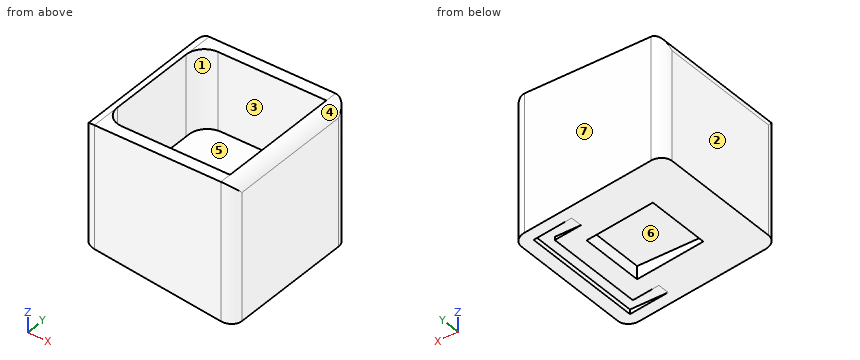
from build123d import *

# Parameters (mm, degrees)
F0_W     = 25
F0_H     = 25
F0_W_2   = 21
F0_H_2   = 21
F1_DEPTH = 23
F0_W_3   = 17
F0_H_3   = 17
F2_DEPTH = 5
F0_W_4   = 11
F0_H_4   = 11
F3_DEPTH = 12
F4_DEPTH = 3
F5_DEPTH = 1
F7_DEPTH = 25
F8_R     = 1.99999
F9_R     = 3


# Not quite as in the source:
# - a fillet or chamfer is up to 0.001 mm smaller than in the source, because OpenCascade refuses the exact size


with BuildPart() as f1:
    # F0 (on Top) → F1 (new body)
    with BuildSketch(Plane.XY):
        with Locations((12.5, -12.5)):
            Rectangle(F0_W, F0_H)
        with Locations((12.5, -12.5)):
            Rectangle(F0_W_2, F0_H_2, mode=Mode.SUBTRACT)
    extrude(amount=F1_DEPTH)

    # F0 (on Top) → F2 (join)
    with BuildSketch(Plane.XY):
        with Locations((12.5, -12.5)):
            Rectangle(F0_W_2, F0_H_2)
        with Locations((12.5, -12.5)):
            Rectangle(F0_W_3, F0_H_3, mode=Mode.SUBTRACT)
    extrude(amount=F2_DEPTH)

    # F0 (on Top) → F3 (join)
    with BuildSketch(Plane.XY):
        with Locations((12.5, -12.5)):
            Rectangle(F0_W_3, F0_H_3)
        with Locations((12.5, -12.5)):
            Rectangle(F0_W_4, F0_H_4, mode=Mode.SUBTRACT)
        with Locations((12.5, -12.5)):
            Rectangle(F0_W_4, F0_H_4)
    extrude(amount=F3_DEPTH)

    # F0 (on Top) → F4 (cut)
    with BuildSketch(Plane.XY):
        with Locations((12.5, -12.5)):
            Rectangle(F0_W_4, F0_H_4)
    extrude(amount=F4_DEPTH, mode=Mode.SUBTRACT)

    # F0 (on Top) → F5 (cut)
    with BuildSketch(Plane.XY):
        with Locations((12.5, -12.5)):
            Rectangle(F0_W_2, F0_H_2)
        with Locations((12.5, -12.5)):
            Rectangle(F0_W_3, F0_H_3, mode=Mode.SUBTRACT)
    extrude(amount=F5_DEPTH, mode=Mode.SUBTRACT)

    # F6 (on face) → F7 (cut, through all)
    with BuildSketch(Plane.XZ.offset(25)):
        Polygon((25, 0), (0, 3), (0, 0), align=None)
    extrude(amount=-F7_DEPTH, mode=Mode.SUBTRACT)

    # F8 (radius 2 in the source; OpenCascade refuses exactly that, so slightly less here)
    f8_edges = [f1.edges().sort_by_distance(p)[0] for p in [
        (25, -25, 11.5),
        (0, -25, 13),
        (0, 0, 13),
        (25, 0, 11.5),
        (0, -12.5, 23),
        (25, -12.5, 23),
    ]]
    fillet(f8_edges, radius=F8_R)

    # F9
    f9_edges = [f1.edges().sort_by_distance(p)[0] for p in [
        (2, -2, 14),
        (4, -4, 8.5),
        (21, -4, 8.5),
        (21, -21, 8.5),
        (4, -21, 8.5),
        (2, -23, 14),
    ]]
    fillet(f9_edges, radius=F9_R)


solid = f1.part
Geometry check sheet. Reference: the model listing, model coordinates, mm. Face numbers are marked on the shaded views. A direction names the side the tool comes from. Round coordinates to 2 decimals unless told otherwise and drop trailing zeros. Order: outer loops, then holes, each group sorted by start corner. A loop starts at its lowest first (then second) coordinate and runs counter-clockwise, first axis right, second up. Notation, with made-up numbers: M 48.5,68 L 77.5,68 A14 cw 77.5,80 Z; hole C -13.5,48 d9. An arc over 180 degrees is marked long. Answer in a Markdown table with one row per item. Add a question column.
Item 1: Sectioned sample at B-B, the plane x = 12.75. Enter the section's corners in (y, z), plus the area to 3 significant figures.
Item 2: Set-up check for the marked faces 5, 6 and 7: record each of +Z, -Z, +X, -X, +Y, -Y from which the full face is reachable in a straight line by a thin tool's end or side.
Item 3: Material ranges on L1, parallel to Y at x = 15.75, z = 7.75; L2, parallel to X at y = -17.5, z = 9.75; L3, parallel to Y at x = 8.5, z = 19, recorded low to high. Write a range as [from, to].
Item 4: Sectioned sample at C-C, the plane z = 19. Enter the section's corners in (x, y).
Item 5: Draft check along X on the marked faces 1, 2, 3 and 4. Enter one of: released by +X, released by -X, zero draft, split by the parting line, or undercut.
Item 6: Sectioned sample at A-A, the plane z = 6.75. Enter the section's corners in (x, y), plus the area to 3 significant figures.
Item 7: Depth check by flat-ended pin: pin 1 Ø3 at (x, y) = (19, -14) entering from -Z. Enter the tip coordinate at first touch or a pass-through.
Filled in:
| question | item | result |
|---|---|---|
| 1 | outline | M -25,1.47 L -18,1.47 L -18,3 L -7,3 L -7,1.47 L 0,1.47 L 0,23 L -2,23 L -2,5 L -4,5 L -4,12 L -21,12 L -21,5 L -23,5 L -23,23 L -25,23 Z |
| 1 | area | 262 mm² |
| 2 | face 5 | +Z |
| 2 | face 6 | -Z |
| 2 | face 7 | +Z, -Z, +X, -X, +Y |
| 3 | L1 | y = [-25, -23], [-21, -4], [-2, 0] |
| 3 | L2 | x = [0, 2], [4, 21], [23, 25] |
| 3 | L3 | y = [-25, -23], [-2, 0] |
| 4 | outline | M 0,-23 A2 ccw 2,-25 L 23,-25 A2 ccw 25,-23 L 25,-2 A2 ccw 23,0 L 2,0 A2 ccw 0,-2 Z; hole M 2,-20 A3 ccw 5,-23 L 23,-23 L 23,-2 L 5,-2 A3 ccw 2,-5 Z |
| 5 | face 1 | undercut |
| 5 | face 2 | released by -X |
| 5 | face 3 | undercut |
| 5 | face 4 | released by +X |
| 6 | outline | M 0,-23 A2 ccw 2,-25 L 23,-25 A2 ccw 25,-23 L 25,-2 A2 ccw 23,0 L 2,0 A2 ccw 0,-2 Z; M 4,-18 A3 ccw 7,-21 L 18,-21 A3 ccw 21,-18 L 21,-7 A3 ccw 18,-4 L 7,-4 A3 ccw 4,-7 Z; hole M 2,-20 A3 ccw 5,-23 L 23,-23 L 23,-2 L 5,-2 A3 ccw 2,-5 Z |
| 6 | area | 466 mm² |
| 7 | pin 1 | stops at z = 0.54 |
